Geometry: final body of the model. Coordinates: model frame, mm. A direction names the side the tool comes from. Round coordinates to 2 decimals unless told otherwise and drop trailing zeros. Order: outer loops, then holes, each group sorted by start corner. A loop starts at its lowest first (then second) coordinate and runs counter-clockwise, first axis right, second up. Notation, with made-up numbers: M -15,46.5 L 36,46.5 A28 cw 36,72.5 Z; hole C 58,4 d11. An arc over 180 degrees is marked long. Return JSON: item names as keys, results as strings. Group by question number.
Q1. Mould query, pull axis X, two halves, no side actions, for faces 4 (the face through (-72.5, 7, 15)), 5 (the face through (-39, -3, -24)), 6 (the face through (-35.77, -1.48, 24.6)). Classes: released by +X, released by -X, zero draft, split by the parting line, or undercut.
Q2. Access query for faces 1 (the face through (-5.062, 42.325, 22.794)), 2 (the face through (-62, 8.824, -18)), 3 (the face through (42.49, -1.48, -23.14)). Directions: +Z, -Z, +X, -X, +Y, -Y. A direction counts if a zero-diameter tool reaches every point of the face in a straight line with its end or side. Return the directions, or none.
Q3. Cut plane B-B on z = 0. Output: boundary loops of the cut face in (x, y), and give its area (3 significant figures).
Q4. Contact query for flat-ended pins moving along their axis: pin 1 (4 mm diameter, centred on x = 14, y = 48, fed in from -Z); pin 2 (8 mm diameter, centred on y = 38.5, z = 0, fed in from +X); pin 3 (2 mm diameter, centred on x = -27, z = -10, fed in from +Y). Output: stop coordinate, or through.
Q5. Cut plane C-C on x = -54. Output: boundary loops of the cut face in (y, z), and give its area (3 significant figures).
Q6. Cut plane A-A on x = 0. Output: boundary loops of the cut face in (y, z), and give its area (3 significant figures).
Q7. Ray query, probe 1 along X at (y, z) = (17.5, -23); probe 2 along Y at (x, z) = (-7.5, -16); probe 3 along Y at (x, z) = (-40, -3). Return the intervals inside material, ascending.
Q8. Cut plane D-D on y = 16. Output: boundary loops of the cut face in (x, z), and give its area (3 significant figures).
```python
from build123d import *

# Parameters (mm, degrees)
SKETCH1_W           = 105
SKETCH1_H           = 53.3
BOSS_EXTRUDE1_DEPTH = 30
SKETCH2_R           = 4.818720667
SKETCH2_W           = 7.589906064
SKETCH2_H           = 7.253051844
BOSS_EXTRUDE2_DEPTH = 20
SKETCH3_R           = 23.34946898
BOSS_EXTRUDE3_DEPTH = 25
SKETCH4_R           = 1.5
BOSS_EXTRUDE4_DEPTH = 3


with BuildPart() as part:
    # Sketch1 → Boss-Extrude1 (new body)
    with BuildSketch(Plane(origin=(0, 0, 0), x_dir=(1, 0, 0), z_dir=(0, 1, 0))):
        Rectangle(SKETCH1_W, SKETCH1_H)
    extrude(amount=BOSS_EXTRUDE1_DEPTH)

    # Sketch2 → Boss-Extrude2 (add)
    with BuildSketch(Plane.ZY.offset(52.5)):
        with Locations((14.56750928, 6.602710937)):
            Circle(SKETCH2_R)
        with Locations((-17.806950585, 5.197359545)):
            Rectangle(SKETCH2_W, SKETCH2_H)
    extrude(amount=BOSS_EXTRUDE2_DEPTH)

    # Sketch3 → Boss-Extrude3 (add)
    with BuildSketch(Plane(origin=(0, 30, 0), x_dir=(1, 0, 0), z_dir=(0, 1, 0))):
        Circle(SKETCH3_R)
    extrude(amount=BOSS_EXTRUDE3_DEPTH)

    # Sketch4 → Boss-Extrude4 (add)
    with BuildSketch(Plane.XZ):
        with Locations((-37.2, 24.15)):
            Circle(SKETCH4_R)
        with Locations((-38.5, -24.15)):
            Circle(SKETCH4_R)
        with Locations((37.7, 24.15)):
            Circle(SKETCH4_R)
        with Locations((43.6, -24.15)):
            Circle(SKETCH4_R)
    extrude(amount=BOSS_EXTRUDE4_DEPTH)


solid = part.part
```
Result sheet:
{
 "1": {"face 4": "released by -X", "face 5": "zero draft", "face 6": "undercut"},
 "2": {"face 1": "+Y", "face 2": "-Z, -X, +Y", "face 3": "-Y"},
 "3": {"outline": "M -52.5,0 L 52.5,0 L 52.5,30 L 23.35,30 L 23.35,55 L -23.35,55 L -23.35,30 L -52.5,30 Z", "area": "4,320 mm²"},
 "4": {"pin 1": "stops at z = -20.03", "pin 2": "stops at x = 23.35", "pin 3": "stops at y = 30"},
 "5": {"outline": "M 1.57,-21.6 L 8.82,-21.6 L 8.82,-14.01 L 1.57,-14.01 Z; C 6.6,14.57 d9.64", "area": "128 mm²"},
 "6": {"outline": "M 0,-26.65 L 30,-26.65 L 30,-23.35 L 55,-23.35 L 55,23.35 L 30,23.35 L 30,26.65 L 0,26.65 Z", "area": "2,770 mm²"},
 "7": {"probe 1": "x = -52.5 to 52.5", "probe 2": "y = 0 to 55", "probe 3": "y = 0 to 30"},
 "8": {"outline": "M -52.5,-26.65 L 52.5,-26.65 L 52.5,26.65 L -52.5,26.65 Z", "area": "5,600 mm²"}
}
